Answer from the drawing. Dimensions are ordinates in mm from the lowest x, y and z of the part. Coordinates: 2 decimals unless noted, no trailing zeros. Write each loop counter-clockwise with the first axis right and the second up, starting at its lowest first coordinate (ties: lowest second). Pieces come first, ordered by that corner, then holes. Notation, with made-up numbers: (-36, 26) - (14, 26) arc R26 cw to (14, 49) - close; hole circle Ø7 at (-28.5, -39). An arc over 180 degrees is marked (long way). Answer as a JSON object with one key per item and string values. Group by question number.
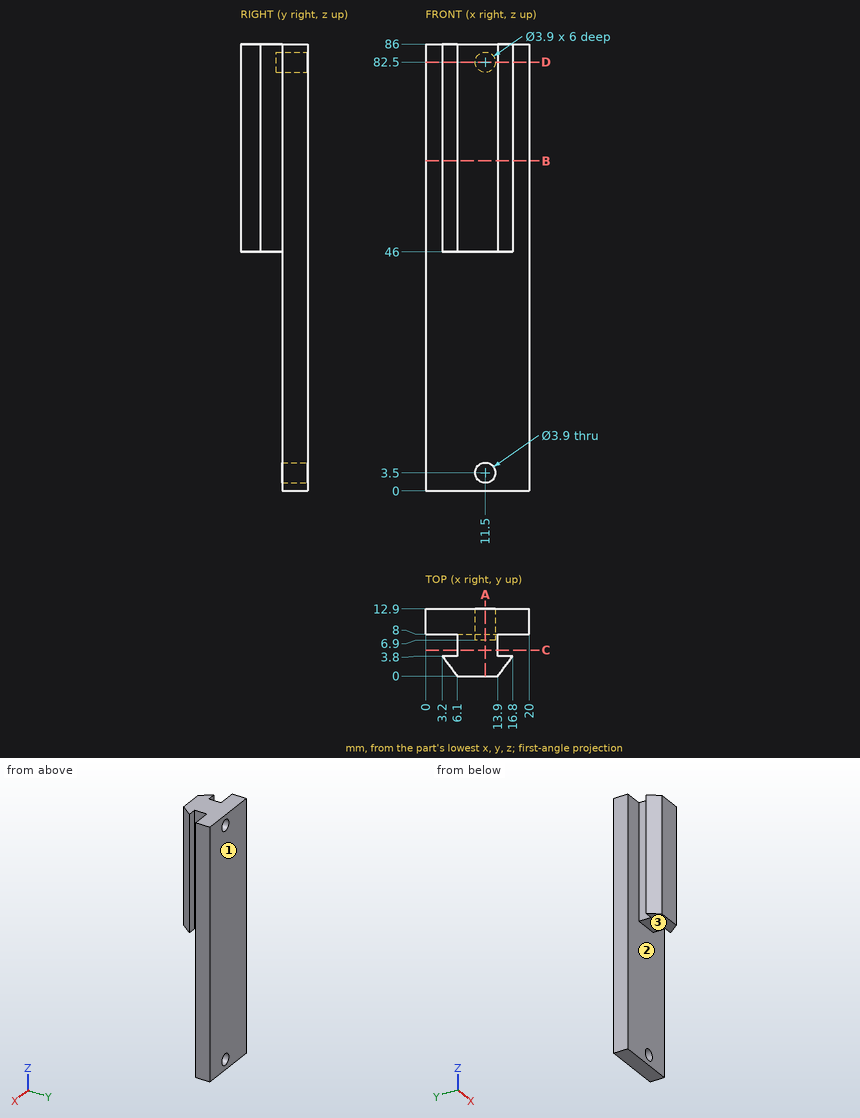
Q1. Section B-B on z = 63.5 is taken. Determine the outline of the cut face in (x, y), plus the area to 3 significant figures.
Q2. For a pull along Y with two mould halves and no side action, classify the marked faces 1, 2 and 3 as +Y half, -Y half, draft (parallel to the pull), parting line (faces both ways), or undercut.
Q3. Consider L1, parallel to Z at x = 11.5, y = 11.2; L2, parallel to X at y = 10.2, z = 82.5; L3, parallel to Y at x = 16, z = 36. Determine where each line is inside the solid, lowest interval first. Write a range as from..to.
Q4. Section C-C on y = 5 is taken. Determine the outline of the cut face in (x, z).
Q5. Section D-D on z = 82.5 is taken. Determine the outline of the cut face in (x, y).
Q6. Section A-A on x = 11.5 is taken. Determine the outline of the cut face in (y, z), plus the area to 3 significant figures.
Q7. Flat-ended cylindrical pins translate along their axes: pin 1 Ø1.2 at (x, z) = (11, 82) entering from +Y; pin 2 Ø4 at (x, z) = (4, 39.5) entering from -Y; pin 3 Ø5 at (y, z) = (3.5, 68) entering from +X. Find the tip coordinate at first contact, or state that the pin passes through.
Numbers:
{
 "1": {"outline": "(0, 8) - (6.1, 8) - (6.1, 3.8) - (3.2, 3.8) - (6.1, 0) - (13.9, 0) - (16.8, 3.8) - (13.9, 3.8) - (13.9, 8) - (20, 8) - (20, 12.9) - (0, 12.9) - close", "area": "171 mm²"},
 "2": {"face 1": "+Y half", "face 2": "undercut", "face 3": "draft"},
 "3": {"L1": "z = 0..1.55, 5.45..80.55, 84.45..86", "L2": "x = 0..9.55, 13.45..20", "L3": "y = 8..12.9"},
 "4": {"outline": "(6.1, 46) - (13.9, 46) - (13.9, 86) - (6.1, 86) - close"},
 "5": {"outline": "(0, 8) - (6.1, 8) - (6.1, 3.8) - (3.2, 3.8) - (6.1, 0) - (13.9, 0) - (16.8, 3.8) - (13.9, 3.8) - (13.9, 8) - (20, 8) - (20, 12.9) - (13.45, 12.9) - (13.45, 6.9) - (9.55, 6.9) - (9.55, 12.9) - (0, 12.9) - close"},
 "6": {"outline": "(0, 46) - (8, 46) - (8, 5.45) - (12.9, 5.45) - (12.9, 80.55) - (6.9, 80.55) - (6.9, 84.45) - (12.9, 84.45) - (12.9, 86) - (0, 86) - close; (8, 0) - (12.9, 0) - (12.9, 1.55) - (8, 1.55) - close", "area": "699 mm²"},
 "7": {"pin 1": "stops at y = 6.9", "pin 2": "stops at y = 8", "pin 3": "stops at x = 16.8"}
}
